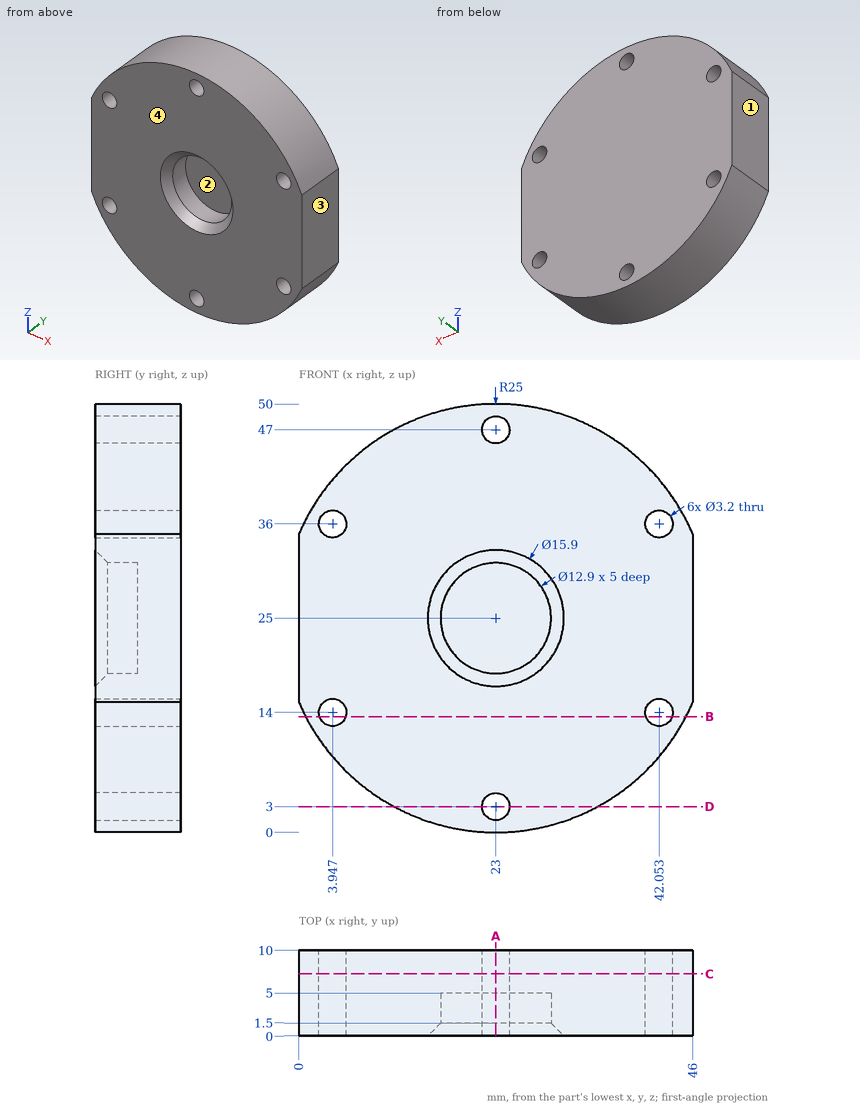
Design review of the part shown in the three views and the two pictorial views. Dimensions are in mm from the part's minimum x, y and z. Give positions to 0.01 mm unless a question says otherwise; leave off trailing zeros. Loops run counter-clockwise (first coordinate to the right, second up) from the corner with the lowest first, then second, coordinate; pieces in that order, holes last. Notation, with made-up numbers: M 23,21.25 L 28,21.25 A24 cw 28,54.25 Z; hole C 83,81.5 d8. An arc over 180 degrees is marked long. Answer as a JSON object with one key per item and string values.
Item 1: We need section A-A (x = 23). State the section outline as (y, z) points, and give its area (3 significant figures).
Output values:
{"outline": "M 0,0 L 10,0 L 10,1.4 L 0,1.4 Z; M 0,4.6 L 10,4.6 L 10,45.4 L 0,45.4 L 0,32.95 L 1.5,31.45 L 5,31.45 L 5,18.55 L 1.5,18.55 L 0,17.05 Z; M 0,48.6 L 10,48.6 L 10,50 L 0,50 Z", "area": "369 mm2"}
Item 2: We need section D-D (z = 3). State the section outline as (x, y) points (1 decimal).
Output values:
{"outline": "M 11.1,0 L 21.4,0 L 21.4,10 L 11.1,10 Z; M 24.6,0 L 34.9,0 L 34.9,10 L 24.6,10 Z"}
Item 3: Mouldability with a two-part tool opening along X and no side actions: class the marked faces 1, 2, 3 and 4 as pulls with the +X half, pulls with the -X half, needs draft (parallel to the pull), parting line crosses it, or undercut.
Output values:
{"face 1": "pulls with the -X half", "face 2": "undercut", "face 3": "pulls with the +X half", "face 4": "needs draft"}
Item 4: Wall thickness on line 1 along X through (y, z) = (3.8, 25); line 2 along X through (y, z) = (2, 14); line 3 along Z through (x, y) = (4, 9.5): over which ranges is each line inside the solid? List them lowest first.
Output values:
{"line 1": "x = 0 to 16.55, 29.45 to 46", "line 2": "x = 0.55 to 2.35, 5.55 to 40.45, 43.65 to 45.45", "line 3": "z = 8.75 to 12.4, 15.6 to 34.4, 37.6 to 41.25"}
Item 5: We need section C-C (y = 7.25). State the section outline as (x, z) points, and give its area (3 significant figures).
Output values:
{"outline": "M 0,15.2 A25 ccw 46,15.2 L 46,34.8 A25 ccw 0,34.8 Z; hole C 3.95,14 d3.2; hole C 3.95,36 d3.2; hole C 23,3 d3.2; hole C 23,47 d3.2; hole C 42.05,14 d3.2; hole C 42.05,36 d3.2", "area": "1,860 mm2"}
Item 6: For P1, Ø10.5, axis at x = 23.5, z = 23.5, coming from the -Y side; P2, Ø3.5, axis at x = 23, z = 47, coming from the -Y side; P3, Ø1, axis at x = 30.5, y = 2.5, coming from the -Z side; P4, Ø7.5, axis at x = 23, z = 25, coming from the -Y side, all flat-tipped, find the tip position at first contact; note any pin that passes through.
Output values:
{"P1": "stops at y = 1.12", "P2": "stops at y = 0", "P3": "stops at z = 1", "P4": "stops at y = 5"}
Item 7: We need section B-B (z = 13.5). State the section outline as (x, y) points, and give its area (3 significant figures).
Output values:
{"outline": "M 0.8,0 L 2.43,0 L 2.43,10 L 0.8,10 Z; M 5.47,0 L 40.53,0 L 40.53,10 L 5.47,10 Z; M 43.57,0 L 45.2,0 L 45.2,10 L 43.57,10 Z", "area": "383 mm2"}
